Could you check a few things on this model? Use its own coordinates, in mm. A direction names the side the tool comes from. Round coordinates to 2 decimals unless told otherwise and drop trailing zeros. Loops run counter-clockwise (first coordinate to the right, second up) from the corner with the lowest first, then second, coordinate; pieces in that order, holes last. Notation, with made-up numbers: (64, 22.5) - (88, 22.5) arc R20 ccw to (88, 37.5) - close; hole circle Ø2 at (64, 34). An arc over 180 degrees is marked (long way). Answer as CSV lines item,"result". Start each with the question number.
1) Which directions (+Z, -Z, +X, -X, +Y, -Y) give clear straight access to the entire face, cutting with the end or side of a thin tool? Please do faces 1 (the face through (1, 4, -10.248)), 2 (the face through (12, 4, 9.752)), 3 (the face through (11, 1, 6.752)), 4 (the face through (18.93, 9.99, -1.12)), 5 (the face through (1, 3, -13)).
2) I'm going to push flat-ended pins straight in: pin 1 Ø1.4 at (x, z) = (3.41, -1.25) entering from +Y; pin 2 Ø0.6 at (x, z) = (10.5, 8.5) entering from +Y; pin 3 Ø1 at (x, z) = (-9.59, -1.25) entering from -Y; pin 4 Ø2.5 at (x, y) = (-13.5, 5) entering from +Z. Where does each tip first touch, or does it pass through?
3) Suppose I cut it at C-C, the plane x = -6. Write out the boundary of the cut face in (y, z).
4) Suppose I cut it at A-A, the plane y = 10.75. Write out the boundary of the cut face in (x, z).
5) Please list where these lines run through material, in increasing order: line 1 along Z through (x, y) = (-15.5, 5.75); line 2 along X through (y, z) = (9.5, -5); line 3 along Y through (x, z) = (-11, 9).
6) Suppose I cut it at D-D, the plane y = 4.5. Write out the boundary of the cut face in (x, z), then the cut area to 3 significant figures.
7) Suppose I cut it at B-B, the plane y = 9. Write out the boundary of the cut face in (x, z), then the cut area to 3 significant figures.
8) We'd pull the mould along Y, two halves only. Please class faces 6 (the face through (12, 4, 7.752)), 7 (the face through (18.887, 6.843, -6.71)), 8 (the face through (-14, 6, 9)): pulls with the +Y half, pulls with the -Y half, needs draft (parallel to the pull), parting line crosses it, or undercut.
```python
from build123d import *

# Parameters (mm, degrees)
CROQUIS1_W              = 39
CROQUIS1_H              = 25
CROQUIS1_R              = 4.000000275
CROQUIS1_R_2            = 0.600000034
CROQUIS1_W_2            = 8
CROQUIS1_H_2            = 6
SALIENTE_EXTRUIR1_DEPTH = 3
SALIENTE_EXTRUIR2_DEPTH = 3
CROQUIS3_W              = 3
CROQUIS3_H              = 25
SALIENTE_EXTRUIR3_DEPTH = 6
CROQUIS4_R              = 1
CORTAR_EXTRUIR1_DEPTH   = 45
CROQUIS5_R              = 1
CORTAR_EXTRUIR2_DEPTH   = 27


with BuildPart() as part:
    # Croquis1 → Saliente-Extruir1 (new body)
    with BuildSketch(Plane(origin=(0, 0, 0), x_dir=(1, 0, 0), z_dir=(0, 1, 0))):
        with Locations((0.907645754, 1.248012912)):
            Rectangle(CROQUIS1_W, CROQUIS1_H)
        with Locations((-3.09235459, 1.24801291)):
            Circle(CROQUIS1_R, mode=Mode.SUBTRACT)
        with Locations((-3.092354224, 7.748013103)):
            Circle(CROQUIS1_R_2, mode=Mode.SUBTRACT)
        with Locations((3.407645945, 1.248012891)):
            Circle(CROQUIS1_R_2, mode=Mode.SUBTRACT)
        with Locations((-3.092354267, -5.251987278)):
            Circle(CROQUIS1_R_2, mode=Mode.SUBTRACT)
        with Locations((-9.592354436, 1.248012934)):
            Circle(CROQUIS1_R_2, mode=Mode.SUBTRACT)
        with Locations((10.907645754, -3.751987088)):
            Rectangle(CROQUIS1_W_2, CROQUIS1_H_2, mode=Mode.SUBTRACT)
        with Locations((10.907645754, 6.248012912)):
            Rectangle(CROQUIS1_W_2, CROQUIS1_H_2, mode=Mode.SUBTRACT)
    extrude(amount=SALIENTE_EXTRUIR1_DEPTH)

    # Croquis2 → Saliente-Extruir2 (add)
    with BuildSketch(Plane(origin=(0, 3, 0), x_dir=(1, 0, 0), z_dir=(0, 1, 0))):
        Polygon((-18.592354246, 13.748012912), (-15.592354246, 13.748012912), (-15.592354246, 12.248012912), (17.407645754, 12.248012912), (17.407645754, 13.748012912), (20.407645754, 13.748012912), (20.407645754, -11.251987088), (17.407645754, -11.251987088), (17.407645754, -9.751987088), (5.907645754, -9.751987088), (5.907645754, -7.751987088), (17.407645754, -7.751987088), (17.407645754, 10.248012912), (-15.592354246, 10.248012912), (-15.592354246, -7.751987088), (-12.092354246, -7.751987088), (-12.092354246, -9.751987088), (-15.592354246, -9.751987088), (-15.592354246, -11.251987088), (-18.592354246, -11.251987088), align=None)
    extrude(amount=SALIENTE_EXTRUIR2_DEPTH)

    # Croquis3 → Saliente-Extruir3 (add)
    with BuildSketch(Plane(origin=(0, 6, 0), x_dir=(1, 0, 0), z_dir=(0, 1, 0))):
        with Locations((-17.092354246, 1.248012912)):
            Rectangle(CROQUIS3_W, CROQUIS3_H)
        with Locations((18.907645754, 1.248012912)):
            Rectangle(CROQUIS3_W, CROQUIS3_H)
    extrude(amount=SALIENTE_EXTRUIR3_DEPTH)

    # Croquis4 → Cortar-Extruir1 (cut)
    with BuildSketch(Plane.ZY.offset(18.592354246)):
        with Locations((-7.248012912, 6)):
            Circle(CROQUIS4_R)
        with Locations((4.751987088, 6)):
            Circle(CROQUIS4_R)
    extrude(amount=-CORTAR_EXTRUIR1_DEPTH, mode=Mode.SUBTRACT)

    # Croquis5 → Cortar-Extruir2 (cut)
    with BuildSketch(Plane(origin=(20.407645754, 0, 0), x_dir=(0, 0, -1), z_dir=(1, 0, 0))):
        with Locations((1.248012912, 9)):
            Circle(CROQUIS5_R)
    extrude(amount=-CORTAR_EXTRUIR2_DEPTH, mode=Mode.SUBTRACT)


solid = part.part
```
Filled sheet:
1,face 1,"+Y"
1,face 2,"+Z, +Y"
1,face 3,"+Y, -Y"
1,face 4,"+X"
1,face 5,"-Z, +Y"
2,pin 1,"y = 3"
2,pin 2,"y = 6"
2,pin 3,"through"
2,pin 4,"z = 9.75"
3,outline,"(0, -13.75) - (3, -13.75) - (3, -12.25) - (6, -12.25) - (6, -10.25) - (3, -10.25) - (3, -3.99) - (0, -3.99) - close; (0, 1.5) - (3, 1.5) - (3, 11.25) - (0, 11.25) - close"
4,outline,"(-18.59, -13.75) - (-15.59, -13.75) - (-15.59, 11.25) - (-18.59, 11.25) - close; (17.41, -13.75) - (20.41, -13.75) - (20.41, 11.25) - (17.41, 11.25) - close"
5,line 1,"-12.25 to -10.25, 7.75 to 9.75"
5,line 2,"-18.59 to -15.59, 17.41 to 20.41"
5,line 3,"0 to 3"
6,outline,"(-18.59, -13.75) - (-15.59, -13.75) - (-15.59, -12.25) - (17.41, -12.25) - (17.41, -13.75) - (20.41, -13.75) - (20.41, 11.25) - (17.41, 11.25) - (17.41, 9.75) - (5.91, 9.75) - (5.91, 7.75) - (17.41, 7.75) - (17.41, -10.25) - (-15.59, -10.25) - (-15.59, 7.75) - (-12.09, 7.75) - (-12.09, 9.75) - (-15.59, 9.75) - (-15.59, 11.25) - (-18.59, 11.25) - close"
6,area,"246 mm²"
7,outline,"(-18.59, -13.75) - (-15.59, -13.75) - (-15.59, 11.25) - (-18.59, 11.25) - close; (17.41, -13.75) - (20.41, -13.75) - (20.41, -2.25) - (17.41, -2.25) - close; (17.41, -0.25) - (20.41, -0.25) - (20.41, 11.25) - (17.41, 11.25) - close"
7,area,"144 mm²"
8,face 6,"needs draft"
8,face 7,"undercut"
8,face 8,"pulls with the +Y half"
